```python
from build123d import *

# Parameters (mm, degrees)
SKETCH2_R           = 2.286
MAIN_DEPTH          = 6.35
SKETCH5_W           = 12.7
SKETCH5_H           = 6.35
SKETCH5_H_2         = 35.219317332
ACRYLIC_JOINT_DEPTH = 123.31992325
SKETCH6_W           = 3.81
SKETCH6_H           = 39.029317332
CUT_EXTRUDE1_DEPTH  = 123.31992325
FILLET4_R           = 3.175


with BuildPart() as part:
    # Sketch2 → Main (new body)
    with BuildSketch(Plane(origin=(0, 0, 0), x_dir=(0, 0, -1), z_dir=(1, 0, 0))):
        Polygon((-67.818, 101.6), (-67.818, 19.812), (-36.068, 19.812), (-29.718, 13.462), (-29.718, 7.9375), (-24.1935, 7.9375), (45.72, 7.9375), (52.07, 7.9375), (52.07, 30.456817332), (-19.073182668, 101.6), (-55.118, 101.6), align=None)
        with Locations((-61.468, 26.162)):
            Circle(SKETCH2_R, mode=Mode.SUBTRACT)
        with Locations((-61.468, 95.25)):
            Circle(SKETCH2_R, mode=Mode.SUBTRACT)
    extrude(amount=MAIN_DEPTH)

    # Sketch5 → Acrylic Joint (cut, through all)
    with BuildSketch(Plane(origin=(6.35, 0, 0), x_dir=(0, 0, -1), z_dir=(1, 0, 0))):
        with Locations((-30.48, 11.1125)):
            Rectangle(SKETCH5_W, SKETCH5_H)
        with Locations((-5.08, 11.1125)):
            Rectangle(SKETCH5_W, SKETCH5_H)
        with Locations((20.32, 11.1125)):
            Rectangle(SKETCH5_W, SKETCH5_H)
        Polygon((16.847841816, 56.698719395), (21.337969877, 61.188847455), (30.318225998, 52.208591334), (25.828097937, 47.718463274), align=None)
        Polygon((-1.112670426, 74.659231637), (3.377457634, 79.149359697), (12.357713756, 70.169103576), (7.867585695, 65.678975516), align=None)
        Polygon((-19.073182668, 92.619743879), (-14.583054608, 97.109871939), (-5.602798487, 88.129615818), (-10.092926547, 83.639487758), align=None)
        with Locations((45.72, 25.547158666)):
            Rectangle(SKETCH5_W, SKETCH5_H_2)
    extrude(amount=-ACRYLIC_JOINT_DEPTH, mode=Mode.SUBTRACT)

    # Sketch6 → Cut-Extrude1 (cut, through all)
    with BuildSketch(Plane(origin=(6.35, 0, 0), x_dir=(0, 0, -1), z_dir=(1, 0, 0))):
        with Locations((37.465, 27.452158666)):
            Rectangle(SKETCH6_W, SKETCH6_H)
    extrude(amount=-CUT_EXTRUDE1_DEPTH, mode=Mode.SUBTRACT)

    # Fillet4
    fillet4_edges = [part.edges().sort_by_distance(p)[0] for p in [
        (3.175, 46.966817332, -35.56),
        (3.175, 19.812, 36.068),
        (3.175, 19.812, 67.818),
        (3.175, 101.6, 67.818),
        (3.175, 101.6, 19.073182668),
    ]]
    fillet(fillet4_edges, radius=FILLET4_R)


solid = part.part
```
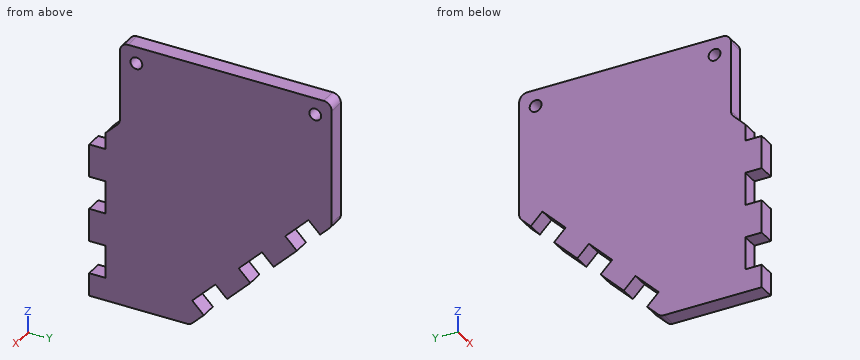
Source: CAD feature listing. Evaluate the final solid. Frame: model axes, mm. Give positions to 0.01 mm unless a question says otherwise; leave off trailing zeros. Loops run counter-clockwise (first coordinate to the right, second up) from the corner with the lowest first, then second, coordinate; pieces in that order, holes last. Notation, with made-up numbers: (50, 53) -> (84, 53) arc R15 cw to (84, 67) -> close; hole circle Ø9 at (40.25, 88.25). An arc over 180 degrees is marked (long way). Use a Markdown table: item, result. Add a question column.
(1) Section query A-A (y = 95.25). Output: boundary loops of the cut face in (x, z).
(2) Section query B-B (z = 54.5). Output: boundary loops of the cut face in (x, y), then the cut area to 3 significant figures.
(3) Section query D-D (y = 16). Output: boundary loops of the cut face in (x, z), then the cut area to 3 significant figures.
(4) First-contact query: pin 1 Ø1.9 at (x, y) = (2, 12) entering from +Z; pin 2 Ø1.9 at (x, z) = (2.5, 7.5) entering from -Y; pin 3 Ø2 at (x, z) = (4, 40.5) entering from -Y. Flat tips, straight axial feed; report the tip coordinate or a pass-through.
(5) Section query C-C (x = 2). Count the separate pieces of the cut face and the enclosed holes in it, then the cut area to 3 significant figures.
(6) Ray query, line 1 (Y direction, x = 4.5, z = 52); line 2 (Y direction, x = 3.5, z = 18.5); line 3 (Z direction, x = 5, y = 68.5). Return the intervals inside material, ascending.
Checked values:
| question | item | result |
|---|---|---|
| 1 | outline | (0, 16.44) -> (6.35, 16.44) -> (6.35, 59.18) -> (0, 59.18) -> close; (0, 63.75) -> (6.35, 63.75) -> (6.35, 67.82) -> (0, 67.82) -> close |
| 2 | outline | (0, 19.81) -> (6.35, 19.81) -> (6.35, 101.6) -> (0, 101.6) -> close |
| 2 | area | 519 mm^2 |
| 3 | outline | (0, -35.56) -> (6.35, -35.56) -> (6.35, 32.26) -> (0, 32.26) -> close |
| 3 | area | 431 mm^2 |
| 4 | pin 1 | z = 24.13 |
| 4 | pin 2 | y = 14.29 |
| 4 | pin 3 | y = 19.81 |
| 5 | separate pieces | 1 |
| 5 | enclosed holes | 2 |
| 5 | area | 7,280 mm^2 |
| 6 | line 1 | 19.81 to 101.6 |
| 6 | line 2 | 7.94 to 92.05, 93.19 to 100.98 |
| 6 | line 3 | -14.03 to -10.69, -5.05 to 67.82 |
